Geometry check sheet. Reference: the model listing, model coordinates, mm. A direction names the side the tool comes from. Coordinates: 2 decimals unless noted, no trailing zeros. Write each loop counter-clockwise with the first axis right and the second up, starting at its lowest first coordinate (ties: lowest second). Pieces come first, ordered by that corner, then holes. Notation, with made-up numbers: (57.25, -5) -> (66.25, -5) arc R6 cw to (66.25, 0) -> close; hole circle Ø3 at (-15.75, 15.25). An arc over 180 degrees is marked (long way). Use a Markdown table: item, result.
```python
from build123d import *

# Parameters (mm, degrees)
PAD_DEPTH    = 250
SKETCH001_W  = 2
SKETCH001_H  = 45
POCKET_DEPTH = 20


with BuildPart() as part:
    # Sketch → Pad (new body)
    with BuildSketch(Plane.XY):
        with BuildLine():
            Line((0, 0), (0, 57))
            Line((0, 57), (38, 57))
            Line((38, 57), (38, 1))
            ThreePointArc((23.5, 10), (29.345332, 3.236924), (38, 1))
            Line((23.5, 10), (16, 10))
            Line((16, 10), (16, 0))
            Line((16, 0), (0, 0))
        make_face()
    extrude(amount=PAD_DEPTH)

    # Sketch001 (on Face3 of Pad) → Pocket (cut)
    with BuildSketch(Plane.YZ.offset(38)):
        with Locations((22, 57.5)):
            Rectangle(SKETCH001_W, SKETCH001_H)
    extrude(amount=-POCKET_DEPTH, mode=Mode.SUBTRACT)


solid = part.part
```
Item 1: Depth check by flat-ended pin: P1, Ø0.6, axis at y = 22.5, z = 59.5, coming from the +X side; P2, Ø12, axis at x = 31.5, z = 46, coming from the -Y side; P3, Ø6, axis at x = 19.5, z = 176, coming from the -Y side. Enter the tip coordinate at first touch or a pass-through.
Answer block:
| item | result |
|---|---|
| P1 | stops at x = 18 |
| P2 | stops at y = 0.98 |
| P3 | stops at y = 10 |
Item 2: Section check A-A on y = 5. Record the boundary of the cut face in (x, z), then the cut area to 3 significant figures.
Answer block:
| item | result |
|---|---|
| outline | (0, 0) -> (16, 0) -> (16, 250) -> (0, 250) -> close; (27.04, 0) -> (38, 0) -> (38, 250) -> (27.04, 250) -> close |
| area | 6,740 mm^2 |
Item 3: Section check B-B on z = 98. Record the boundary of the cut face in (x, y).
Answer block:
| item | result |
|---|---|
| outline | (0, 0) -> (16, 0) -> (16, 10) -> (23.5, 10) arc R15 ccw to (38, 1) -> (38, 57) -> (0, 57) -> close |
Item 4: Mould release check, pull along X, two halves, no side actions. Record for faces 4 (the flat face through (38, 29, 123)), 5 (the flat face through (19, 29, 250)), 6 (the flat face through (16, 5, 123)): +X half, -X half, draft (parallel to the pull), parting line (faces both ways), or undercut.
Answer block:
| item | result |
|---|---|
| face 4 | +X half |
| face 5 | draft |
| face 6 | undercut |
Item 5: Tool access check on faces 1 (the flat face through (0, 28, 123)), 2 (the flat face through (28, 23, 57)), 3 (the flat face through (20, 10, 123)). Record the directions out of +Z, -Z, +X, -X, +Y, -Y that give a thin tool (end or side, any length) a straight path to the whole face; none if there is none.
Answer block:
| item | result |
|---|---|
| face 1 | +Z, -Z, -X, +Y, -Y |
| face 2 | +X |
| face 3 | +Z, -Z, -Y |
Item 6: Section check C-C on x = 28. Record the boundary of the cut face in (y, z), then the cut area to 3 significant figures.
Answer block:
| item | result |
|---|---|
| outline | (4.18, 0) -> (57, 0) -> (57, 250) -> (4.18, 250) -> close; hole (21, 35) -> (23, 35) -> (23, 80) -> (21, 80) -> close |
| area | 13,100 mm^2 |
Item 7: Thickness scan on L1, parallel to Y at x = 20.5, z = 70.5; L2, parallel to Y at x = 17.5, z = 28.5; L3, parallel to Z at x = 28.5, y = 22. Record the ranges inside material, lowest first. Write a range as [from, to].
Answer block:
| item | result |
|---|---|
| L1 | y = [10, 21], [23, 57] |
| L2 | y = [10, 57] |
| L3 | z = [0, 35], [80, 250] |
Item 8: Section check D-D on z = 41.5. Record the boundary of the cut face in (x, y).
Answer block:
| item | result |
|---|---|
| outline | (0, 0) -> (16, 0) -> (16, 10) -> (23.5, 10) arc R15 ccw to (38, 1) -> (38, 21) -> (18, 21) -> (18, 23) -> (38, 23) -> (38, 57) -> (0, 57) -> close |
